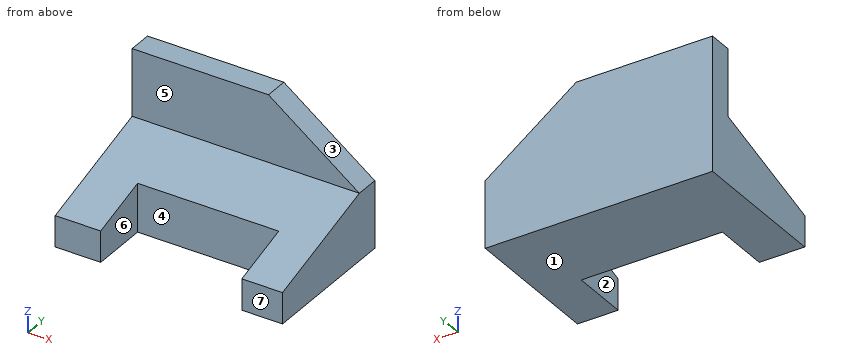
from build123d import *

# Parameters (mm, degrees)
F1_DEPTH = 47.5
F2_W     = 59
F2_H     = 24
F3_DEPTH = 25
F5_DEPTH = 10


with BuildPart() as f1:
    # F0 (on Right) → F1 (new body, symmetric)
    with BuildSketch(Plane.YZ):
        Polygon((-30, 13), (-30, 0), (30, 0), (30, 56), (20, 56), (20, 28), align=None)
    extrude(amount=F1_DEPTH, both=True)

    # F2 (on Top) → F3 (cut)
    with BuildSketch(Plane.XY):
        with Locations((1, -18)):
            Rectangle(F2_W, F2_H)
    extrude(amount=F3_DEPTH, mode=Mode.SUBTRACT)

    # F4 (on face) → F5 (cut, through all)
    with BuildSketch(Plane.XZ.offset(-20)):
        Polygon((47.5, 56), (9.5, 56), (47.5, 28), align=None)
    extrude(amount=-F5_DEPTH, mode=Mode.SUBTRACT)


solid = f1.part
Build history of the part. All positions in model axes, mm. Face numbers are marked on the shaded views. A direction names the side the tool comes from. Coordinates: 2 decimals unless noted, no trailing zeros. Order: outer loops, then holes, each group sorted by start corner. A loop starts at its lowest first (then second) coordinate and runs counter-clockwise, first axis right, second up. Notation, with made-up numbers: (-6, 45) - (45, 45) arc R16 ccw to (45, 68) - close; hole circle Ø2 at (26, 20). An arc over 180 degrees is marked (long way). Put each result on its own line as item: value.
1. Saw through at B-B (x = -7.5). Write the cut outline in (y, z).
Answer sheet:
outline: (-6, 0) - (30, 0) - (30, 56) - (20, 56) - (20, 28) - (-6, 20.2) - close
2. Probe line 1 along Y through (x, z) = (-2.5, 8); line 2 along Y through (x, z) = (20, 38.5); line 3 along Z through (x, y) = (26, 4). List the from-to ranges inside material, lowest first. Write a range as [from, to].
Answer sheet:
line 1: y = [-6, 30]
line 2: y = [20, 30]
line 3: z = [0, 23.2]
3. Saw through at C-C (y = 24.5). Write the cut outline in (x, z).
Answer sheet:
outline: (-47.5, 0) - (47.5, 0) - (47.5, 28) - (9.5, 56) - (-47.5, 56) - close
4. Saw through at A-A (y = -15). Write the cut outline in (x, z).
Answer sheet:
outline: (-47.5, 0) - (-28.5, 0) - (-28.5, 17.5) - (-47.5, 17.5) - close; (30.5, 0) - (47.5, 0) - (47.5, 17.5) - (30.5, 17.5) - close
5. Drop flat-ended pins along their axis: P1, Ø10, axis at x = 10, z = 12, coming from the -Y side; P2, Ø12, axis at x = 1.5, y = -10.5, coming from the +Z side; P3, Ø8.5, axis at x = -14.5, z = 38.5, coming from the -Y side. Give the stop position or say it passes through.
Answer sheet:
P1: stops at y = -6
P2: stops at z = 20.65
P3: stops at y = 20
6. Tool access for the marked faces 5, 6 and 7: list every direction of +Z, -Z, +X, -X, +Y, -Y with a clear straight run to the whole face (end or side of a thin tool).
Answer sheet:
face 5: +Z, +X, -X, -Y
face 6: +Z, -Z, -Y
face 7: +Z, -Z, +X, -X, -Y
7. Saw through at D-D (z = 25). Write the cut outline in (x, y).
Answer sheet:
outline: (-47.5, 10) - (47.5, 10) - (47.5, 30) - (-47.5, 30) - close
8. Pull direction X, two halves, no side cores. Call the marked faces 1, 2, 3 and 4: pulls with the +X half, pulls with the -X half, needs draft (parallel to the pull), parting line crosses it, or undercut.
Answer sheet:
face 1: needs draft
face 2: undercut
face 3: pulls with the +X half
face 4: undercut
